from build123d import *


with BuildPart() as f1:
    # F0 (on Front) → F1 (revolve)
    with BuildSketch(Plane.XZ):
        with BuildLine():
            Line((0, 31), (0, 0))
            Line((0, 0), (88, 0))
            Line((88, 0), (88, 15))
            Line((88, 15), (85, 15))
            Line((85, 15), (85, 20))
            Line((85, 20), (68, 20))
            Line((68, 20), (68, 31))
            Line((68, 31), (56, 31))
            ThreePointArc((56, 31), (50, 25), (44, 31))
            Line((44, 31), (0, 31))
        make_face()
    revolve(axis=Axis((54.523584, 0, 0), (1, 0, 0)))

    # F2 (on Front) → F3 (revolve, cut)
    with BuildSketch(Plane.XZ):
        Polygon((0, 25), (0, 0), (135.937035, 0), (135.937035, 6), (30, 6), (30, 16), (22, 16), (22, 20.5), (16.5, 20.5), (16.5, 12.5), (13.5, 12.5), (13.5, 16), (1.5, 16), (1.5, 25), align=None)
    revolve(axis=Axis((-19.679806, 0, 0), (-1, 0, 0)), mode=Mode.SUBTRACT)


solid = f1.part
CAD build for the part. Positions are in the model's coordinates, mm. A direction names the side the tool comes from. Round coordinates to 2 decimals unless told otherwise and drop trailing zeros. Write each loop counter-clockwise with the first axis right and the second up, starting at its lowest first coordinate (ties: lowest second). Pieces come first, ordered by that corner, then holes.
(1) Slice it at B-B, the plane x = 11.5. Write the cut outline in (y, z).
(2) Mould opens along Y. For faces 1 (the face through (76.381, 19.524, -4.336)), 2 (the face through (85, -15, -3)), 3 (the face through (25.94, -15.62, -3.47)) say: pulls with the +Y half, pulls with the -Y half, needs draft (parallel to the pull), parting line crosses it, or undercut.
(3) 3-axis set-ups, long thin cutter, end or side, ignore diameter. For faces 4 (the face through (0, -14, -21)), 5 (the face through (0.74, 7.509, 23.846)), 6 (the face through (30, 0, -7)), 7 (the face through (88, 6.5, 0.2)), 8 (the face through (68, 20.2, 0.4)): which of +Z, -Z, +X, -X, +Y, -Y reach the whole face in a straight line?
(4) Probe line 1 along X through (y, z) = (-20, 9.5); line 2 along X through (y, z) = (-6.5, -1.5); line 3 along Y through (x, z) = (15.65, 0). List the from-to ranges inside material, lowest first.
(5) Slice it at A-A, the plane x = 31. Write the cut outline in (y, z), and give its area (3 significant figures).
(6) Drop flat-ended pins along their axis: P1, Ø1, axis at y = -23.5, z = -1.5, coming from the -X side; P2, Ø19, axis at y = 0, z = 0, coming from the -X side; P3, Ø9.5, axis at y = -3, z = 7.5, coming from the -X side. Give the stop position or say it passes through.
From the geometry:
1. outline: circle Ø62 at (0, 0); hole circle Ø32 at (0, 0)
2. face 1: parting line crosses it
2. face 2: needs draft
2. face 3: undercut
3. face 4: +Z, -Z, -X, +Y, -Y
3. face 5: -X
3. face 6: none
3. face 7: +Z, -Z, +X, +Y, -Y
3. face 8: +X
4. line 1: x = 1.5 to 68
4. line 2: x = 30 to 88
4. line 3: y = -31 to -12.5, 12.5 to 31
5. outline: circle Ø62 at (0, 0); hole circle Ø12 at (0, 0)
5. area: 2,910 mm2
6. P1: stops at x = 1.5
6. P2: stops at x = 30
6. P3: stops at x = 13.5
